Verification items for this drawing (mm, ordinates from the low corner). A direction names the side the tool comes from. Coordinates: 2 decimals unless noted, no trailing zeros. Loops run counter-clockwise (first coordinate to the right, second up) from the corner with the lowest first, then second, coordinate; pieces in that order, holes last. Notation, with made-up numbers: (2, -20.5) - (8, -20.5) arc R25 ccw to (8, 13.5) - close; hole circle Ø4 at (-3.75, 10.5). An arc over 180 degrees is marked (long way). Write each question's results on one line, items separated by ' | '. Start each with the question number.
(1) Sectioned sample at C-C (x = 33.5). Enter the section's corners in (y, z) (1 decimal).
(2) Sectioned sample at A-A (z = 38.5). Enter the section's corners in (x, y) (1 decimal).
(3) Sectioned sample at D-D (z = 7). Enter the section's corners in (x, y) (1 decimal), plus the area to 3 significant figures.
(4) Material ranges on probe 1 along X at (y, z) = (32, 37) (1 decimal); probe 2 along Z at (x, y) = (32.5, 12.5); probe 3 along X at (y, z) = (35, 17), recorded low to high.
(5) Access from +Z, -Z, +X, -X, +Y, -Y to the whole of each face (thin tool, end or side, straight path). Record for the marked faces 1, 2, 3, 4 and 5.
(6) Go/stop test with flat-tipped pins: pin 1 Ø4 at (y, z) = (26.5, 33.5) entering from -X; pin 2 Ø2 at (y, z) = (29.5, 20) entering from -X; pin 3 Ø6 at (x, y) = (4.5, 5.5) entering from +Z; pin 4 Ø3.5 at (x, z) = (33.5, 7) entering from +Y (1 decimal). Record where each tip stops, or that it passes through.
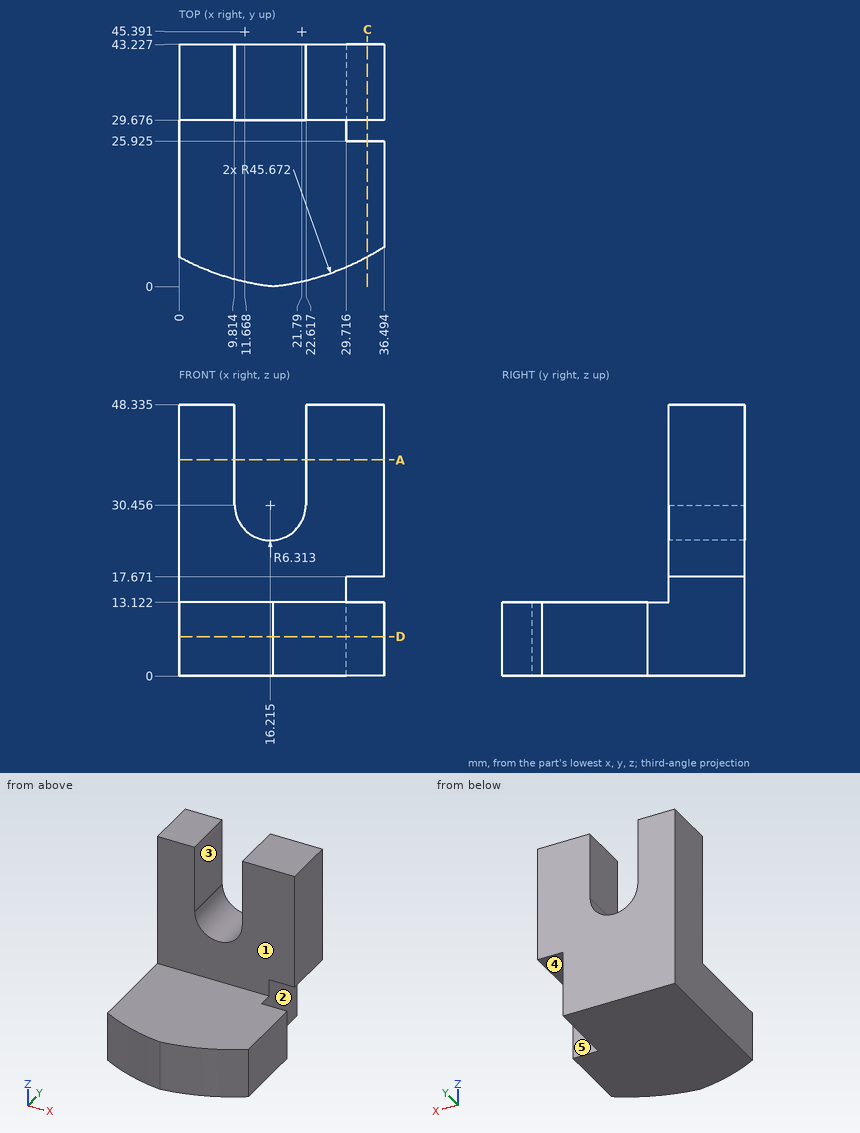
Outcome:
1) outline: (5.3, 0) - (25.9, 0) - (25.9, 13.1) - (5.3, 13.1) - close; (29.7, 17.7) - (43.2, 17.7) - (43.2, 48.3) - (29.7, 48.3) - close
2) outline: (0, 29.7) - (9.8, 29.7) - (9.8, 43.2) - (0, 43.2) - close; (22.6, 29.7) - (36.5, 29.7) - (36.5, 43.2) - (22.6, 43.2) - close
3) outline: (0, 5.3) arc R45.7 ccw to (16.7, 0) arc R45.7 ccw to (36.5, 7.1) - (36.5, 25.9) - (29.7, 25.9) - (29.7, 43.2) - (0, 43.2) - close | area: 1,370 mm2
4) probe 1: x = 0 to 9.8, 22.6 to 36.5 | probe 2: z = 0 to 13.12 | probe 3: x = 0 to 29.72
5) face 1: +Z, +X, -X, -Y | face 2: -Z, +X, +Y | face 3: +Z, +Y, -Y | face 4: -Z, +X, +Y, -Y | face 5: +Z, -Z, +X, +Y
6) pin 1: passes through | pin 2: stops at x = 0 | pin 3: stops at z = 13.12 | pin 4: stops at y = 25.9
